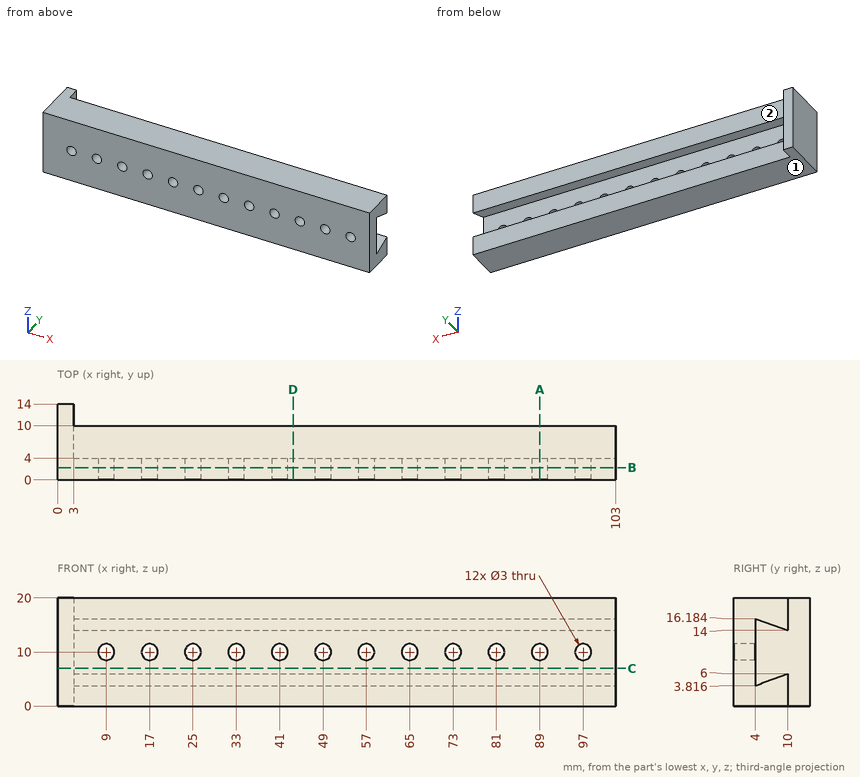
Study the drawing (mm; zero at the part's minimum x, y, z) and answer. A direction names the side the tool comes from. Round coordinates to 2 decimals unless told otherwise and drop trailing zeros. Order: outer loops, then holes, each group sorted by start corner. A loop starts at its lowest first (then second) coordinate and runs counter-clockwise, first axis right, second up. Notation, with made-up numbers: (18, -20) -> (43, -20) arc R20 cw to (43, 4) -> close; hole circle Ø6 at (-33.5, -29). An arc over 180 degrees is marked (long way). Write each question's results on one line, items separated by ' | '. Start each with the question number.
Q1. Find section A-A (x = 89). Determine the outline of the cut face in (y, z), then the cut area to 3 significant figures.
Q2. Find section D-D (x = 43.5). Determine the outline of the cut face in (y, z).
Q3. Find section C-C (z = 7). Determine the outline of the cut face in (x, y), then the cut area to 3 significant figures.
Q4. Find section B-B (y = 2.25). Give the number of separate pieces and of enclosed holes in the cut face, then the cut area to 3 significant figures.
Q5. Straight lines are drawn through the part: probe 1 along Z at (x, y) = (57, 2.35); probe 2 along Y at (x, z) = (37, 17.5); probe 3 along Z at (x, y) = (14, 7.25). For each, find the intervals that lie inside material, in ascending order. Write a range as from..to.
Q6. Each of these flat-tipped pins is pushed along its axis until it touches: pin 1 (2 mm diameter, centred on x = 67, z = 16.5, fed in from +Y); pin 2 (4 mm diameter, centred on x = 65, z = 10, fed in from +Y). Where does it stop, or does it pass through?
Q7. Which of the six approach directions +Z, -Z, +X, -X, +Y, -Y give full straight-line access (tool end or side, diameter ignored) to the marked faces 1 and 2?
Worked answers:
1) outline: (0, 0) -> (10, 0) -> (10, 6) -> (4, 3.82) -> (4, 8.5) -> (0, 8.5) -> close; (0, 11.5) -> (4, 11.5) -> (4, 16.18) -> (10, 14) -> (10, 20) -> (0, 20) -> close | area: 127 mm2
2) outline: (0, 0) -> (10, 0) -> (10, 6) -> (4, 3.82) -> (4, 16.18) -> (10, 14) -> (10, 20) -> (0, 20) -> close
3) outline: (0, 0) -> (103, 0) -> (103, 4) -> (3, 4) -> (3, 14) -> (0, 14) -> close | area: 442 mm2
4) separate pieces: 1 | enclosed holes: 12 | area: 1,980 mm2
5) probe 1: z = 0..8.5, 11.5..20 | probe 2: y = 0..10 | probe 3: z = 0..5, 15..20
6) pin 1: stops at y = 10 | pin 2: stops at y = 4
7) face 1: -Z, +X, -X, +Y, -Y | face 2: +Z, -Z, +X, +Y
